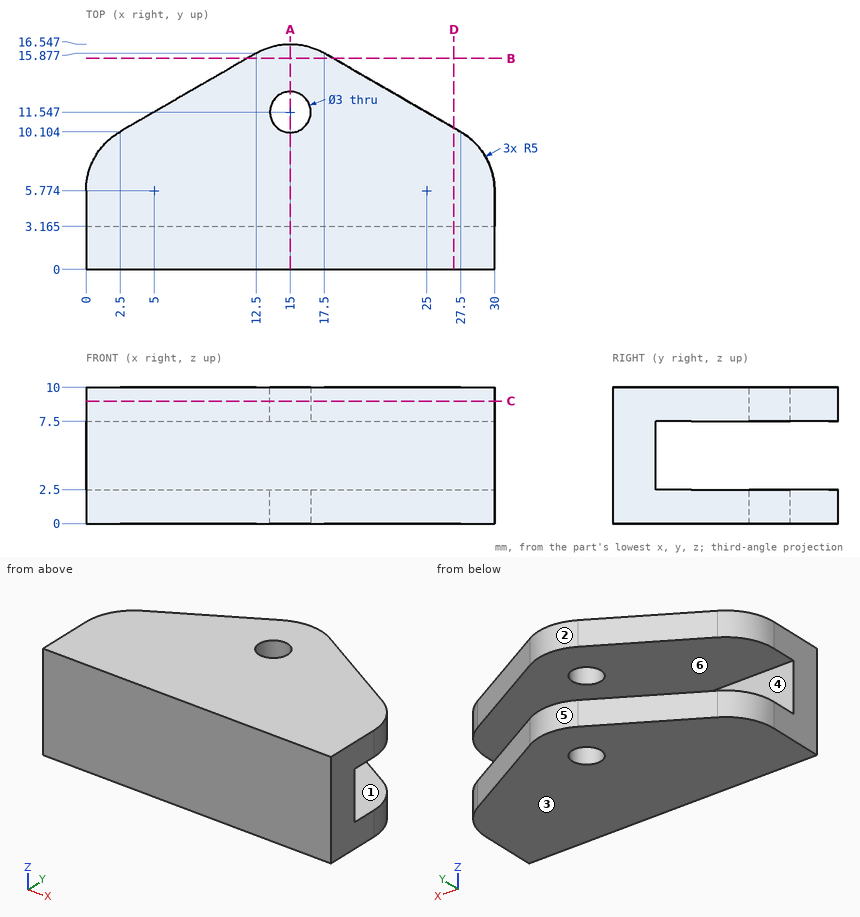
Here's the drawing with two shaded views (mm, measured from the low corner). I have some questions. A direction names the side the tool comes from. Round coordinates to 2 decimals unless told otherwise and drop trailing zeros. Loops run counter-clockwise (first coordinate to the right, second up) from the corner with the lowest first, then second, coordinate; pieces in that order, holes last.
Item 1: Suppose I cut it at C-C, the plane z = 9. Write out the boundary of the cut face in (x, y).
Item 2: Will these pins go through, and if not, where does the flat tip stop? pin 1 Ø2.5 at (x, y) = (15, 11.55) entering from -Z; pin 2 Ø2 at (x, z) = (8, 4) entering from -Y; pin 3 Ø2.5 at (x, z) = (12.5, 5) entering from +Y (1 decimal).
Item 3: If we mould it in two halves opening along Z, with no side actions, what happens to the marked faces 3, 4, 5 and 6? For each: +Z half, -Z half, draft (parallel to the pull), parting line (faces both ways), or undercut.
Item 4: Suppose I cut it at B-B, the plane y = 15.5. Write out the boundary of the cut face in (x, z).
Item 5: Suppose I cut it at D-D, the plane x = 27. Write out the boundary of the cut face in (y, z) (1 decimal).
Item 6: Please list where these lines run through material, in increasing order: L1, parallel to Y at x = 15, z = 8.4; L2, parallel to Z at x = 21.5, y = 7; L3, parallel to Y at x = 11.5, z = 5.5 (1 decimal).
Item 7: Suppose I cut it at A-A, the plane x = 15. Write out the boundary of the cut face in (y, z) (1 decimal).
Item 8: Which directions (+Z, -Z, +X, -X, +Y, -Y) give clear straight access to the entire face, cutting with the end or side of a thin tool? Please do the marked faces 1 and 2.
Reported:
1. outline: (0, 0) - (30, 0) - (30, 5.77) arc R5 ccw to (27.5, 10.1) - (17.5, 15.88) arc R5 ccw to (12.5, 15.88) - (2.5, 10.1) arc R5 ccw to (0, 5.77) - close; hole circle Ø3 at (15, 11.55)
2. pin 1: passes through
2. pin 2: stops at y = 0
2. pin 3: stops at y = 3.2
3. face 3: -Z half
3. face 4: undercut
3. face 5: draft
3. face 6: undercut
4. outline: (11.85, 0) - (18.15, 0) - (18.15, 2.5) - (11.85, 2.5) - close; (11.85, 7.5) - (18.15, 7.5) - (18.15, 10) - (11.85, 10) - close
5. outline: (0, 0) - (10.4, 0) - (10.4, 2.5) - (3.2, 2.5) - (3.2, 7.5) - (10.4, 7.5) - (10.4, 10) - (0, 10) - close
6. L1: y = 0 to 10.05, 13.05 to 16.55
6. L2: z = 0 to 2.5, 7.5 to 10
6. L3: y = 0 to 3.2
7. outline: (0, 0) - (10, 0) - (10, 2.5) - (3.2, 2.5) - (3.2, 7.5) - (10, 7.5) - (10, 10) - (0, 10) - close; (13, 0) - (16.5, 0) - (16.5, 2.5) - (13, 2.5) - close; (13, 7.5) - (16.5, 7.5) - (16.5, 10) - (13, 10) - close
8. face 1: +X, -X, +Y
8. face 2: +Z, -Z, +Y
